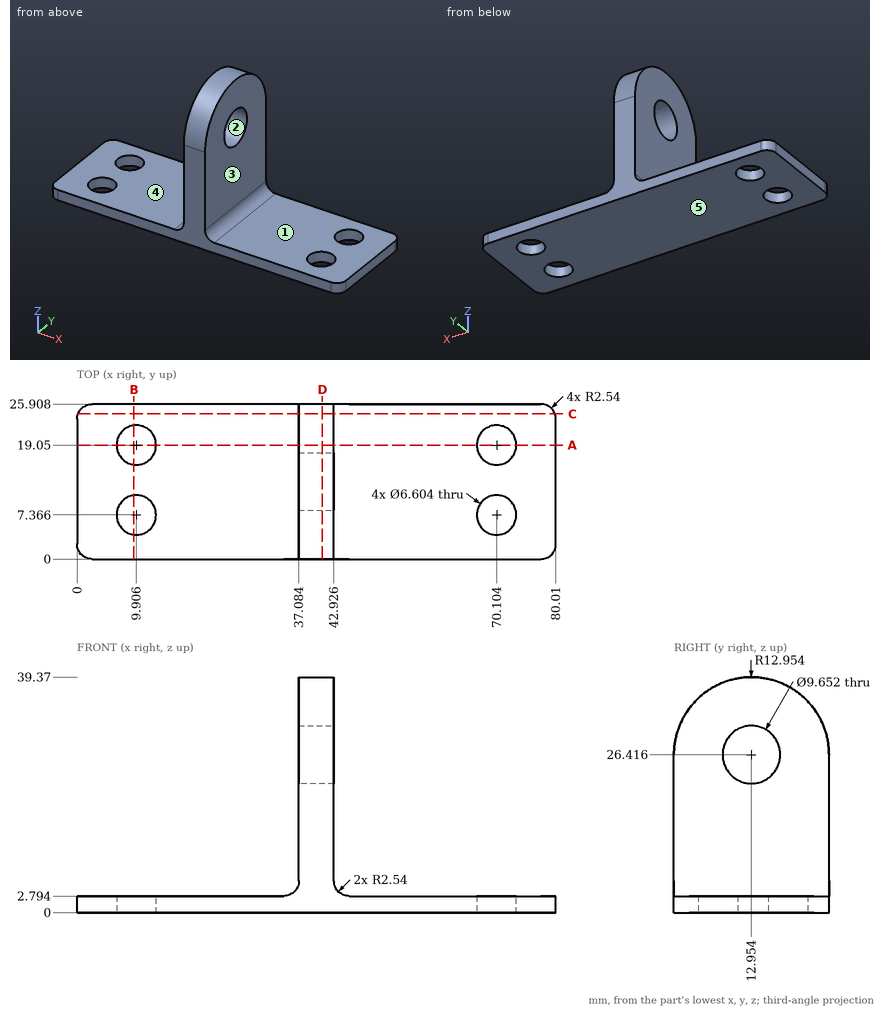
Study the drawing (mm; zero at the part's minimum x, y, z) and answer. A direction names the side the tool comes from. Coordinates: 2 decimals unless noted, no trailing zeros. Write each loop counter-clockwise with the first axis right and the second up, starting at its lowest first coordinate (ties: lowest second). Pieces come first, ordered by that corner, then holes.
Q1. Section B-B, the plane x = 9.5 is taken. Write down the section's boundary in (y, z), then the cut area to 3 significant figures.
Returned:
outline: (0, 0) - (4.09, 0) - (4.09, 2.79) - (0, 2.79) - close; (10.64, 0) - (15.77, 0) - (15.77, 2.79) - (10.64, 2.79) - close; (22.33, 0) - (25.91, 0) - (25.91, 2.79) - (22.33, 2.79) - close
area: 35.8 mm2
Q2. Section A-A, the plane y = 19.05 is taken. Write down the section's boundary in (x, z), then the cut area to 3 significant figures.
Returned:
outline: (0, 0) - (6.6, 0) - (6.6, 2.79) - (0, 2.79) - close; (13.21, 0) - (66.8, 0) - (66.8, 2.79) - (45.47, 2.79) arc R2.54 cw to (42.93, 5.33) - (42.93, 37.85) - (37.08, 37.85) - (37.08, 5.33) arc R2.54 cw to (34.54, 2.79) - (13.21, 2.79) - close; (73.41, 0) - (80.01, 0) - (80.01, 2.79) - (73.41, 2.79) - close
area: 394 mm2
Q3. Find the intervals of material crossed by line 1 along X through (y, z) = (4.25, 18); line 2 along Z through (x, y) = (22, 6.5); line 3 along Z through (x, y) = (37.5, 10), in increasing order.
Returned:
line 1: x = 37.08 to 42.93
line 2: z = 0 to 2.79
line 3: z = 0 to 22.6, 30.23 to 39.03
Q4. Which of the six approach directions +Z, -Z, +X, -X, +Y, -Y give full straight-line access (tool end or side, diameter ignored) to the marked faces 4 and 5?
Returned:
face 4: +Z, -X, +Y, -Y
face 5: -Z, +X, -X, +Y, -Y
Q5. Given P1, Ø1.5, axis at x = 39.5, y = 4.5, coming from the +Z side; P2, Ø2, axis at y = 7, z = 14, coming from the -X side; P3, Ø12, axis at y = 13.5, z = 5.5, coming from the +X side; P4, Ø1, axis at x = 13.5, y = 12, coming from the +Z side, each flat-ended and moving along its own axis, determine where each tip first touches the part or whether it passes through.
Returned:
P1: stops at z = 36.83
P2: stops at x = 37.08
P3: stops at x = 80.01
P4: stops at z = 2.79
Q6. Section C-C, the plane y = 24.25 is taken. Write down the section's boundary in (x, z), then the cut area to 3 significant figures.
Returned:
outline: (0.16, 0) - (79.85, 0) - (79.85, 2.79) - (45.47, 2.79) arc R2.54 cw to (42.93, 5.33) - (42.93, 32.76) - (37.08, 32.76) - (37.08, 5.33) arc R2.54 cw to (34.54, 2.79) - (0.16, 2.79) - close
area: 400 mm2
Q7. Section D-D, the plane x = 41 is taken. Write down the section's boundary in (y, z), then the cut area to 3 significant figures.
Returned:
outline: (0, 0) - (25.91, 0) - (25.91, 26.42) arc R12.95 ccw to (0, 26.42) - close; hole circle Ø9.65 at (12.95, 26.42)
area: 875 mm2
Q8. The mould has two halves that part along Z. Classify the marked faces 1, 2 and 3: released by +Z, released by -Z, zero draft, split by the parting line, or undercut.
Returned:
face 1: released by +Z
face 2: undercut
face 3: zero draft
